```python
from build123d import *

# Parameters (mm, degrees)
SKETCH1_W           = 22
SKETCH1_H           = 82.75
SKETCH1_R           = 3.1
BOSS_EXTRUDE1_DEPTH = 30
SKETCH2_W           = 22
SKETCH2_H           = 82.75
BOSS_EXTRUDE2_DEPTH = 5
SKETCH3_W           = 16
SKETCH3_H           = 35
SKETCH3_R           = 3.1
SKETCH3_W_2         = 22
SKETCH3_H_2         = 14
BOSS_EXTRUDE3_DEPTH = 5


with BuildPart() as part:
    # Sketch1 → Boss-Extrude1 (new body)
    with BuildSketch(Plane.XY):
        with Locations((0, 7.844654309)):
            Rectangle(SKETCH1_W, SKETCH1_H)
        with Locations((0, 35.719654309)):
            Circle(SKETCH1_R, mode=Mode.SUBTRACT)
        with Locations((0, 7.719654309)):
            Circle(SKETCH1_R, mode=Mode.SUBTRACT)
    extrude(amount=BOSS_EXTRUDE1_DEPTH)

    # Sketch2 → Boss-Extrude2 (add)
    with BuildSketch(Plane.XY.offset(30)):
        with Locations((0, 7.844654309)):
            Rectangle(SKETCH2_W, SKETCH2_H)
    extrude(amount=BOSS_EXTRUDE2_DEPTH)

    # Sketch3 → Boss-Extrude3 (add)
    with BuildSketch(Plane.XZ.offset(33.530345691)):
        with Locations((-19, 17.5)):
            Rectangle(SKETCH3_W, SKETCH3_H)
        with Locations((-19, 26)):
            Circle(SKETCH3_R, mode=Mode.SUBTRACT)
        with Locations((-19, 9)):
            Circle(SKETCH3_R, mode=Mode.SUBTRACT)
        with Locations((0, -7)):
            Rectangle(SKETCH3_W_2, SKETCH3_H_2)
        with Locations((0, -7)):
            Circle(SKETCH3_R, mode=Mode.SUBTRACT)
    extrude(amount=-BOSS_EXTRUDE3_DEPTH)


solid = part.part
```
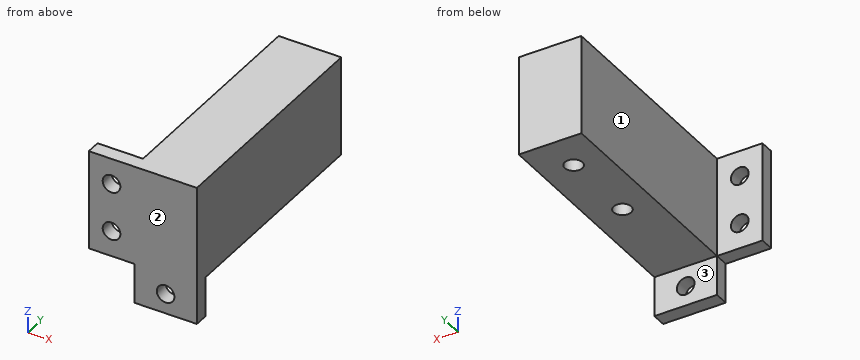
Geometry check sheet. Reference: the model listing, model coordinates, mm. Face numbers are marked on the shaded views. A direction names the side the tool comes from. Coordinates: 2 decimals unless noted, no trailing zeros. Write each loop counter-clockwise with the first axis right and the second up, starting at its lowest first coordinate (ties: lowest second). Pieces come first, ordered by that corner, then holes. Notation, with made-up numbers: M -21,87.25 L 36,87.25 A17 ccw 36,109.25 Z; hole C -6,32 d5. An arc over 180 degrees is marked long. Answer as a JSON object with one key per item and string values.
1. Go/stop test with flat-tipped pins: pin 1 Ø10 at (x, y) = (-11, -1) entering from -Z; pin 2 Ø1.5 at (y, z) = (36.5, 6.5) entering from -X; pin 3 Ø3.5 at (x, y) = (0, 35.72) entering from -Z. Record where each tip stops, or that it passes through.
Answers below:
{"pin 1": "stops at z = 0", "pin 2": "stops at x = -11", "pin 3": "stops at z = 30"}
2. Tool access check on the marked faces 1, 2 and 3. Record the directions out of +Z, -Z, +X, -X, +Y, -Y that give a thin tool (end or side, any length) a straight path to the whole face; none if there is none.
Answers below:
{"face 1": "+Z, -Z, -X, +Y", "face 2": "+Z, -Z, +X, -X, -Y", "face 3": "-Z, +X, -X, +Y"}
3. Section check D-D, the plane z = 17.5. Enter the section's corners in (x, y), plus the area to 3 significant figures.
Answers below:
{"outline": "M -27,-33.53 L 11,-33.53 L 11,49.22 L -11,49.22 L -11,-28.53 L -27,-28.53 Z; hole C 0,7.72 d6.2; hole C 0,35.72 d6.2", "area": "1,840 mm²"}
4. Scan lines: L1, parallel to Y at x = 0, z = 18; L2, parallel to Z at x = 0, y = -30.5; L3, parallel to Y at x = -0.5, z = 18. Record each from-to range of solid material in increasing order.
Answers below:
{"L1": "y = -33.53 to 4.62, 10.82 to 32.62, 38.82 to 49.22", "L2": "z = -14 to -10.1, -3.9 to 35", "L3": "y = -33.53 to 4.66, 10.78 to 32.66, 38.78 to 49.22"}
5. Section check A-A, the plane x = -19. Enter the section's corners in (y, z), plus the area to 3 significant figures.
Answers below:
{"outline": "M -33.53,0 L -28.53,0 L -28.53,5.9 L -33.53,5.9 Z; M -33.53,12.1 L -28.53,12.1 L -28.53,22.9 L -33.53,22.9 Z; M -33.53,29.1 L -28.53,29.1 L -28.53,35 L -33.53,35 Z", "area": "113 mm²"}
6. Section check B-B, the plane z = 27.5. Enter the section's corners in (x, y).
Answers below:
{"outline": "M -27,-33.53 L -21.71,-33.53 L -21.71,-28.53 L -27,-28.53 Z; M -16.29,-33.53 L 11,-33.53 L 11,49.22 L -11,49.22 L -11,-28.53 L -16.29,-28.53 Z; hole C 0,7.72 d6.2; hole C 0,35.72 d6.2"}
7. Section check C-C, the plane z = -7. Enter the section's corners in (x, y).
Answers below:
{"outline": "M -11,-33.53 L -3.1,-33.53 L -3.1,-28.53 L -11,-28.53 Z; M 3.1,-33.53 L 11,-33.53 L 11,-28.53 L 3.1,-28.53 Z"}
